The listing builds one solid part. Answer for the finished solid, in the listing's coordinates (mm). Face numbers are marked on the shaded views. Give positions to 0.01 mm unless a question says otherwise; leave off trailing zeros. Write each loop counter-clockwise with the first axis right and the second up, starting at its lowest first coordinate (ties: lowest second). Pieces come first, ordered by that corner, then holes. Notation, with made-up numbers: M 61,21.5 L 103,21.5 A13 ccw 103,38.5 Z; hole C -16.5,40 d10. An arc over 180 degrees is marked long. Return JSON: item names as keys, results as strings.
Autodesk Inventor part; units mm, degrees
ref_plane "Work Plane1" through (0, 4.5, 0) normal (0, 1, 0) x (-1, 0, 0)
ref_plane "Work Plane2" through (11, 0, 0) normal (1, 0, 0) x (0, 1, 0)
ref_plane "Work Plane3" through (-11, 0, 0) normal (1, 0, 0) x (0, 1, 0)
sketch "Sketch1" plane through (0, 0, 0) normal (0, 1, 0) x (-1, 0, 0)
  line L0 (-20, 59.5) -> (20, 59.5)
  line L1 (20, 59.5) -> (20, -59.5)
  line L2 (20, -59.5) -> (-20, -59.5)
  line L3 (-20, -59.5) -> (-20, 59.5)
  line L4 (-20, 59.5) -> (20, -59.5) construction
  line L5 (20, 59.5) -> (-20, -59.5) construction
  point P0 (0, 0)
  dimension "d0" = 40
  dimension "d1" = 119
extrude "Extrusion1" add sketch "Sketch1" along normal blind 10
sketch "Sketch2" plane through (0, 10, 0) normal (0, 1, 0) x (1, 0, 0)
  line L0 (-16, -41) -> (-6, -41)
  line L1 (-6, -41) -> (-6, 41)
  line L2 (-6, 41) -> (-16, 41)
  line L3 (-16, 41) -> (-16, -41)
  line L4 (-16, -41) -> (-6, 41) construction
  line L5 (-6, -41) -> (-16, 41) construction
  line L6 (16, -41) -> (6, -41)
  line L7 (6, -41) -> (6, 41)
  line L8 (6, 41) -> (16, 41)
  line L9 (16, 41) -> (16, -41)
  line L10 (16, -41) -> (6, 41) construction
  line L11 (6, -41) -> (16, 41) construction
  line L12 (-6, -41) -> (6, -41)
  line L13 (6, -41) -> (6, 41)
  line L14 (6, 41) -> (-6, 41)
  line L15 (-6, 41) -> (-6, -41)
  line L16 (-6, -41) -> (6, 41) construction
  line L17 (6, -41) -> (-6, 41) construction
  point P0 (0, 0)
  point P1 (-11, 0)
  point P2 (11, 0)
  dimension "d4" = 10
  dimension "d5" = 82
  dimension "d6" = 11
  dimension "d7" = 0
  dimension "d8" = 10
  dimension "d9" = 82
  dimension "d10" = 11
  dimension "d21" = 12
  dimension "d22" = 82
extrude "Extrusion3" cut sketch "Sketch2" against normal blind 6
sketch "Sketch3" plane through (0, 4, 0) normal (0, 1, 0) x (1, 0, 0)
  line L0 (-6, -6) -> (6, -6)
  line L1 (6, -6) -> (6, 6)
  line L2 (6, 6) -> (-6, 6)
  line L3 (-6, 6) -> (-6, -6)
  line L4 (-6, -6) -> (6, 6) construction
  line L5 (6, -6) -> (-6, 6) construction
  point P0 (0, 0)
  dimension "d35" = 12
  dimension "d36" = 12
extrude "Extrusion4" cut sketch "Sketch3" against normal blind 6
ref_plane "Work Plane1" through (0, 4.5, 0) normal (0, 1, 0) x (-1, 0, 0)
ref_plane "Work Plane2" through (11, 0, 0) normal (1, 0, 0) x (0, 1, 0)
ref_plane "Work Plane3" through (-11, 0, 0) normal (1, 0, 0) x (0, 1, 0)
ref_plane "Work Plane7" through (-6, 4, -41) normal (0, 0, 1) x (1, 0, 0)
sketch "Sketch6" plane through (-6, 4, -41) normal (0, 0, 1) x (1, 0, 0)
  circle A0 centre (-5, 3) radius 1.5
  line L0 (0, 6) -> (0, 0)
  line L1 (-10, 6) -> (22, 6)
  line L2 (-10, 6) -> (-10, 0)
  point P0 (6, -4)
  point P1 (-9, 6)
  dimension "d42" = 3
  dimension "d44" = 3
  dimension "d112" = 5
ref_plane "Work Plane4" through (7, 4, -40) normal (0, 0, 1) x (1, 0, 0)
sketch "Sketch7" plane through (7, 4, -40) normal (0, 0, 1) x (1, 0, 0)
  circle A0 centre (4, 3) radius 1.5
  line L0 (0, 6) -> (8, 6)
  line L1 (9, 0) -> (9, 6)
  point P0 (-7, -4)
  dimension "d45" = 3
  dimension "d46" = 3
  dimension "d47" = 5
hole "Hole1" at (-11, 7, -41) direction (0, 0, -1) diameter 3 end through all
hole "Hole2" at (11, 7, -40) direction (0, 0, -1) diameter 3 end through all
ref_plane "Work Plane6" through (-6, 4, 41) normal (0, 0, -1) x (-1, 0, 0)
sketch "Sketch8" plane through (-6, 4, 41) normal (0, 0, -1) x (-1, 0, 0)
  circle A0 centre (5, 3) radius 1.5
  line L0 (-22, 6) -> (10, 6)
  line L1 (10, 0) -> (10, 6)
  point P0 (-6, -4)
  point P1 (0, 6)
  point P2 (9, 6)
  dimension "d62" = 3
  dimension "d63" = 3
  dimension "d64" = 5
ref_plane "Work Plane5" through (7, 4, 40) normal (0, 0, -1) x (-1, 0, 0)
sketch "Sketch9" plane through (7, 4, 40) normal (0, 0, -1) x (-1, 0, 0)
  circle A0 centre (-4, 3) radius 1.5
  line L0 (-8, 6) -> (0, 6)
  line L1 (-9, 6) -> (-9, 0)
  point P0 (7, -4)
  dimension "d65" = 3
  dimension "d66" = 3
  dimension "d67" = 5
hole "Hole3" at (-11, 7, 41) direction (0, 0, 1) diameter 3 end through all
hole "Hole4" at (11, 7, 40) direction (0, 0, 1) diameter 3 end through all
sketch "Sketch10" plane through (-20, 0, 59.5) normal (0, 0, 1) x (1, 0, 0)
  circle A0 centre (20, 5) radius 3.25
  line L0 (40, 0) -> (40, 10)
  point P0 (20, 0)
  dimension "d92" = 6.5
  dimension "d93" = 5
  dimension "d94" = 20
hole "Hole5" at (0, 5, 59.5) direction (0, 0, -1) diameter 6.5 depth 18.5
sketch "Sketch11" plane through (20, 0, -59.5) normal (0, 0, -1) x (-1, 0, 0)
  circle A0 centre (20, 5) radius 3.25
  line L0 (40, 0) -> (0, 0)
  line L1 (40, 0) -> (40, 10)
  point P0 (20, 0)
  dimension "d102" = 6.5
  dimension "d103" = 5
  dimension "d104" = 20
hole "Hole6" at (0, 5, -59.5) direction (0, 0, 1) diameter 6 depth 18 tip angle 118
sketch "Sketch12" plane through (0, 10, 0) normal (0, 1, 0) x (1, 0, 0)
  line L0 (-17.5, -41) -> (-16, -41)
  line L1 (-16, -41) -> (-16, 41)
  line L2 (-16, 41) -> (-17.5, 41)
  line L3 (-17.5, 41) -> (-17.5, -41)
  line L4 (-17.5, -41) -> (-16, 41) construction
  line L5 (-16, -41) -> (-17.5, 41) construction
  line L6 (-17.5, -42.5) -> (16, -42.5)
  line L7 (16, -42.5) -> (16, -41)
  line L8 (16, -41) -> (-17.5, -41)
  line L9 (-17.5, -41) -> (-17.5, -42.5)
  line L10 (-17.5, -42.5) -> (16, -41) construction
  line L11 (16, -42.5) -> (-17.5, -41) construction
  point P0 (0, 0)
  point P1 (-16.75, 0)
  point P2 (-0.75, -41.75)
  dimension "d113" = 1.5
  dimension "d114" = 82
  dimension "d115" = 16
  dimension "d116" = 33.5
  dimension "d117" = 1.5
  dimension "d118" = 0
  dimension "d128" = 0.75
extrude "Extrusion7" cut sketch "Sketch12" against normal blind 4
thread "Thread5"
thread "Thread6"
properties part number "BottomSupportPlate"
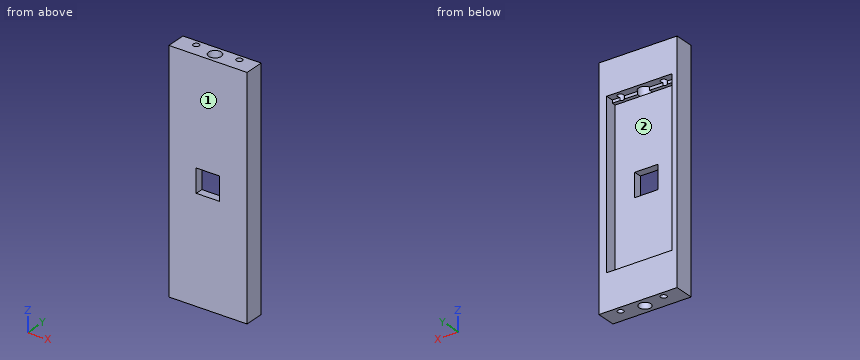
Item 1: A cutting plane is placed at B-B, the plane z = 33.5. Write down the section's boundary in (x, y), plus the area to 3 significant figures.
Geometry results:
{"outline": "M -20,0 L 20,0 L 20,10 L 16,10 L 16,4 L -16,4 L -16,6 L -17.5,6 L -17.5,10 L -20,10 Z", "area": "202 mm2"}
Item 2: A cutting plane is placed at A-A, the plane x = -11. Write down the section's boundary in (y, z), plus the area to 3 significant figures.
Geometry results:
{"outline": "M 0,-59.5 L 5.5,-59.5 L 5.5,-41 L 4,-41 L 4,41 L 5.5,41 L 5.5,59.5 L 0,59.5 Z; M 8.5,-59.5 L 10,-59.5 L 10,-41 L 8.5,-41 Z; M 8.5,42.5 L 10,42.5 L 10,59.5 L 8.5,59.5 Z", "area": "585 mm2"}
Item 3: Determine the mould class of the marked faces 1 and 2 for opening direction Z: +Z half, -Z half, draft (parallel to the pull), parting line (faces both ways), or undercut.
Geometry results:
{"face 1": "draft", "face 2": "undercut"}
Item 4: Find the intervals of material crossed by line 1 (Z direction, x = 6.5, y = 7.75); line 2 (Z direction, x = -1, y = 1); line 3 (X direction, y = 6.75, z = 7), in increasing order.
Geometry results:
{"line 1": "z = -59.5 to -41, 42.5 to 59.5", "line 2": "z = -59.5 to -6, 6 to 59.5", "line 3": "x = -20 to -17.5, 16 to 20"}
Item 5: Given pin 1 Ø0.8 at (x, z) = (6.5, 42) entering from +Y; pin 2 Ø10 at (x, z) = (11.5, -17.5) entering from +Y; pin 3 Ø6 at (x, y) = (0, 5) entering from +Z; pin 4 Ø1 at (x, z) = (-6, 8) entering from +Y, each flat-ended and moving along its own axis, determine where each tip first touches the part or whether it passes through.
Geometry results:
{"pin 1": "stops at y = 6", "pin 2": "stops at y = 10", "pin 3": "stops at z = 41", "pin 4": "stops at y = 4"}
